from build123d import *

# Parameters (mm, degrees)
SKETCH_1_R               = 13.85
EXTRUDE_1_DEPTH          = 37.8
FILLET_1_R               = 1
SKETCH_2_R               = 5
EXTRUDE_2_DEPTH          = 2.6
FILLET_2_R               = 1
SKETCH_3_R               = 1.15
EXTRUDE_3_DEPTH          = 13.8
FILLET_3_R               = 0.5
SKETCH_5_R               = 1.5
CUT_EXTRUDE_1_DEPTH      = 6
EXTRUDE_START            = 2.6
SKETCH_6_R               = 5
EXTRUDE_4_DEPTH          = 2.6
FILLET_4_R               = 1
SKETCH_7_W               = 2.8
SKETCH_7_H               = 0.4
EXTRUDE_5_DEPTH          = 6.9
FILLET_5_R               = 1
CUT_EXTRUDE_3_DEPTH      = 58.630590859
EXTRUDE_7_DEPTH          = 30
CUT_EXTRUDE_2_DEPTH      = 58.630590859
CUT_EXTRUDE_2_DEPTH_BACK = 58.630590859
SKETCH_9_R               = 10
EXTRUDE_6_DEPTH          = 20


with BuildPart() as part:
    # ｽｹｯﾁ1 → ﾎﾞｽ - 押し出し1 (new body)
    with BuildSketch(Plane.XY):
        Circle(SKETCH_1_R)
    extrude(amount=EXTRUDE_1_DEPTH)

    # ﾌｨﾚｯﾄ1
    fillet_1_edges = [part.edges().sort_by_distance(p)[0] for p in [
        (-13.85, 0, 37.8),
    ]]
    fillet(fillet_1_edges, radius=FILLET_1_R)

    # ｽｹｯﾁ2 → ﾎﾞｽ - 押し出し2 (add)
    with BuildSketch(Plane.XY.offset(37.8)):
        Circle(SKETCH_2_R)
    extrude(amount=EXTRUDE_2_DEPTH)

    # ﾌｨﾚｯﾄ2
    fillet_2_edges = [part.edges().sort_by_distance(p)[0] for p in [
        (-5, 0, 40.4),
    ]]
    fillet(fillet_2_edges, radius=FILLET_2_R)

    # ｽｹｯﾁ3 → ﾎﾞｽ - 押し出し3 (add)
    with BuildSketch(Plane.XY.offset(40.4)):
        with Locations(Location((0, 0, 0), (0, 0, 180))):
            Circle(SKETCH_3_R)
    extrude(amount=EXTRUDE_3_DEPTH)

    # ﾌｨﾚｯﾄ3
    fillet_3_edges = [part.edges().sort_by_distance(p)[0] for p in [
        (1.15, 0, 54.2),
    ]]
    fillet(fillet_3_edges, radius=FILLET_3_R)

    # ｽｹｯﾁ5 → ｶｯﾄ - 押し出し1 (cut)
    with BuildSketch(Plane.XY.offset(37.8)):
        with Locations((-0.41868765, 7.989036278)):
            Circle(SKETCH_5_R)
        with Locations((0.41868765, -7.989036278)):
            Circle(SKETCH_5_R)
        with BuildLine():
            ThreePointArc((7.990545371, 5.138208314), (6.35674076, 7.059875842), (4.274821243, 8.483861346))
            ThreePointArc((4.274821243, 8.483861346), (2.260292413, 7.819276067), (2.924877693, 5.804747237))
            ThreePointArc((2.924877693, 5.804747237), (4.349348941, 4.830441366), (5.467215254, 3.515616215))
            ThreePointArc((5.467215254, 3.515616215), (7.540176362, 3.065247206), (7.990545371, 5.138208314))
        make_face()
        with BuildLine():
            ThreePointArc((5.138208314, -7.990545371), (7.059875842, -6.35674076), (8.483861346, -4.274821243))
            ThreePointArc((8.483861346, -4.274821243), (7.819276067, -2.260292413), (5.804747237, -2.924877693))
            ThreePointArc((5.804747237, -2.924877693), (4.830441366, -4.349348941), (3.515616215, -5.467215254))
            ThreePointArc((3.515616215, -5.467215254), (3.065247206, -7.540176362), (5.138208314, -7.990545371))
        make_face()
        with BuildLine():
            ThreePointArc((-7.990545371, -5.138208314), (-6.35674076, -7.059875842), (-4.274821243, -8.483861346))
            ThreePointArc((-4.274821243, -8.483861346), (-2.260292413, -7.819276067), (-2.924877693, -5.804747237))
            ThreePointArc((-2.924877693, -5.804747237), (-4.349348941, -4.830441366), (-5.467215254, -3.515616215))
            ThreePointArc((-5.467215254, -3.515616215), (-7.540176362, -3.065247206), (-7.990545371, -5.138208314))
        make_face()
        with BuildLine():
            ThreePointArc((-5.138208314, 7.990545371), (-7.059875842, 6.35674076), (-8.483861346, 4.274821243))
            ThreePointArc((-8.483861346, 4.274821243), (-7.819276067, 2.260292413), (-5.804747237, 2.924877693))
            ThreePointArc((-5.804747237, 2.924877693), (-4.830441366, 4.349348941), (-3.515616215, 5.467215254))
            ThreePointArc((-3.515616215, 5.467215254), (-3.065247206, 7.540176362), (-5.138208314, 7.990545371))
        make_face()
    extrude(amount=-CUT_EXTRUDE_1_DEPTH, mode=Mode.SUBTRACT)

    # ｽｹｯﾁ6 → ﾎﾞｽ - 押し出し4 (add)
    with BuildSketch(Plane(origin=(0, 0, 0), x_dir=(-1, 0, 0), z_dir=(0, 0, -1)).offset(EXTRUDE_START)):
        with Locations(Location((0, 0, 0), (0, 0, 180))):
            Circle(SKETCH_6_R)
    extrude(amount=-EXTRUDE_4_DEPTH)

    # ﾌｨﾚｯﾄ4
    fillet_4_edges = [part.edges().sort_by_distance(p)[0] for p in [
        (-5, 0, -2.6),
    ]]
    fillet(fillet_4_edges, radius=FILLET_4_R)

    # ｽｹｯﾁ7 → ﾎﾞｽ - 押し出し5 (add)
    with BuildSketch(Plane(origin=(0, 0, 0), x_dir=(-1, 0, 0), z_dir=(0, 0, -1))):
        with Locations((0, 11.5)):
            Rectangle(SKETCH_7_W, SKETCH_7_H)
        with Locations((0, -11.5)):
            Rectangle(SKETCH_7_W, SKETCH_7_H)
    extrude(amount=EXTRUDE_5_DEPTH)

    # ﾌｨﾚｯﾄ5
    fillet_5_edges = [part.edges().sort_by_distance(p)[0] for p in [
        (-1.4, -11.5, -6.9),
        (1.4, -11.5, -6.9),
        (-1.4, 11.5, -6.9),
        (1.4, 11.5, -6.9),
    ]]
    fillet(fillet_5_edges, radius=FILLET_5_R)

    # ｽｹｯﾁ10 → ｶｯﾄ - 押し出し3 (cut, through all)
    with BuildSketch(Plane(origin=(0, 0, 0), x_dir=(0, 0, -1), z_dir=(1, 0, 0))):
        Polygon((-26.8, 5), (-20.8, 5), (-17.8, 3.5), (-17.8, 2), (-26.8, 2), align=None)
        Polygon((-26.8, -2), (-17.8, -2), (-17.8, -3.5), (-20.8, -5), (-26.8, -5), align=None)
    extrude(amount=-CUT_EXTRUDE_3_DEPTH, mode=Mode.SUBTRACT)

    # ｽｹｯﾁ11 → ﾎﾞｽ - 押し出し7 (add)
    with BuildSketch(Plane(origin=(0, 0, 0), x_dir=(-1, 0, 0), z_dir=(0, 0, -1))):
        with BuildLine():
            Line((-13.704834913, 2), (-2, 13.704834913))
            ThreePointArc((-2, 13.704834913), (0, 13.85), (2, 13.704834913))
            Line((2, 13.704834913), (13.704834913, 2))
            ThreePointArc((13.704834913, 2), (13.85, 0), (13.704834913, -2))
            Line((13.704834913, -2), (2, -13.704834913))
            ThreePointArc((2, -13.704834913), (0, -13.85), (-2, -13.704834913))
            Line((-2, -13.704834913), (-13.704834913, -2))
            ThreePointArc((-13.704834913, -2), (-13.85, 0), (-13.704834913, 2))
        make_face()
    extrude(amount=-EXTRUDE_7_DEPTH)

    # ｽｹｯﾁ8 → ｶｯﾄ - 押し出し2 (cut, two sides: drawn at the far end of the back side and taken through both)
    with BuildSketch(Plane(origin=(0, 0, 0), x_dir=(0, 0, -1), z_dir=(1, 0, 0)).offset(-CUT_EXTRUDE_2_DEPTH_BACK)):
        with BuildLine():
            Line((-8, 4), (-8, -4))
            ThreePointArc((-8, -4), (-10, -6), (-12, -4))
            Line((-12, -4), (-12, 4))
            ThreePointArc((-12, 4), (-10, 6), (-8, 4))
        make_face()
    extrude(amount=CUT_EXTRUDE_2_DEPTH + CUT_EXTRUDE_2_DEPTH_BACK, mode=Mode.SUBTRACT)

    # ｽｹｯﾁ9 → ﾎﾞｽ - 押し出し6 (add)
    with BuildSketch(Plane(origin=(0, 0, 0), x_dir=(-1, 0, 0), z_dir=(0, 0, -1))):
        Circle(SKETCH_9_R)
    extrude(amount=-EXTRUDE_6_DEPTH)


solid = part.part
For this review, take the finished solid that the model builds, in its own axes (mm). A direction names the side the tool comes from. Coordinates: 2 decimals unless noted, no trailing zeros. Loops run counter-clockwise (first coordinate to the right, second up) from the corner with the lowest first, then second, coordinate; pieces in that order, holes last. Notation, with made-up numbers: (-35.5, -5.75) - (-8.5, -5.75) arc R31 cw to (-8.5, 22.25) - close; hole circle Ø5 at (21.25, 31.5). An arc over 180 degrees is marked (long way). Use a Markdown table: item, result. Add a question column.
Item 1: Mouldability with a two-part tool opening along Z and no side actions: class faces 6 (the face through (-11, -6, 10)), 7 (the face through (-7.849, 2.275, 34.842)), 8 (the face through (6, -5, 31.8)) as pulls with the +Z half, pulls with the -Z half, needs draft (parallel to the pull), parting line crosses it, or undercut.
Item 2: We need section B-B (z = 10). Give the boundary of the cut face in (x, y).
Item 3: We need section C-C (z = 28.5). Give the boundary of the cut face in (x, y), and give its area (3 significant figures).
Item 4: Insertion check: pin 1 Ø1.5 at (x, y) = (-7.5, -5) entering from +Z; pin 2 Ø4 at (x, y) = (-4.5, 3) entering from -Z; pin 3 Ø2.5 at (x, z) = (-12, 24.5) entering from -Y. Each pin has a flat end and moves straight along its axis. Give the tip position at first contact, or say it passes through.
Item 5: For line 1 (Y direction, x = 6.5, z = 32.5); line 2 (X direction, y = 5, z = 37); line 3 (X direction, y = -8.5, z = 35), list the stretches that pass through material, from the lowest coordinate up.
Item 6: Tool access review of faces 1 (the face through (-13, 4, 26.8)), 2 (the face through (0, -11.7, -3)), 3 (the face through (0.39, 9.25, 34.84)), 4 (the face through (11, 0, 8)), 5 (the face through (0, 11.7, -3)): name each direction out of +Z, -Z, +X, -X, +Y, -Y from which nothing blocks a thin tool from reaching the whole face with its end or side.
Results list:
| question | item | result |
|---|---|---|
| 1 | face 6 | undercut |
| 1 | face 7 | needs draft |
| 1 | face 8 | pulls with the +Z half |
| 2 | outline | (-12.48, -6) arc R13.85 ccw to (12.48, -6) - (8, -6) arc R10 ccw to (8, 6) - (12.48, 6) arc R13.85 ccw to (-12.48, 6) - (-8, 6) arc R10 ccw to (-8, -6) - close |
| 3 | outline | circle Ø27.7 at (0, 0) |
| 3 | area | 603 mm^2 |
| 4 | pin 1 | stops at z = 37.8 |
| 4 | pin 2 | stops at z = -2.6 |
| 4 | pin 3 | stops at y = -8.73 |
| 5 | line 1 | y = -12.23 to -6.93, -2.25 to 2.84, 6.93 to 12.23 |
| 5 | line 2 | x = -12.89 to -8.08, -4.15 to 4.15, 8.07 to 12.89 |
| 5 | line 3 | x = -10.93 to -4.24, -2.96 to -0.99, 1.83 to 10.93 |
| 6 | face 1 | -X |
| 6 | face 2 | -Z, +X, -X, -Y |
| 6 | face 3 | +Z |
| 6 | face 4 | +X |
| 6 | face 5 | -Z, +X, -X, +Y |
